Can you work these out from the model? Positions are in its coordinate system, mm. A direction names the side the tool comes from. Coordinates: 2 decimals unless noted, no trailing zeros. Order: outer loops, then holes, each group sorted by start corner. A loop starts at its lowest first (then second) coordinate and runs counter-clockwise, first axis right, second up. Notation, with made-up numbers: (-32, 55.25) -> (-26, 55.25) arc R22 ccw to (-26, 86.25) -> close; hole circle Ø11 at (2.5, -33). An arc over 180 degrees is marked (long way). Answer as a JSON object with one key per item and string values. Group by question number.
(1) Which directions (+Z, -Z, +X, -X, +Y, -Y) give clear straight access to the entire face, cutting with the end or side of a thin tool? Please do faces 5 (the cylindrical face through (-3, 0, 6)), 6 (the flat face through (5, 0, 4)), 7 (the flat face through (3, 1.5, 1)).
(2) For pin 1 (1 mm diameter, centred on x = 2, y = -1, fed in from +Z), with a flat end and sliding along its axis, tell me the tip position at first contact or that it passes through.
(3) If we mould it in two halves opening along X, with no side actions, what happens to faces 1 (the flat face through (2, 4, 4)), 2 (the flat face through (0, 0, 3)), 3 (the flat face through (-4, 0, 4)), 4 (the flat face through (9, 0, 6))? For each: pulls with the +X half, pulls with the -X half, needs draft (parallel to the pull), parting line crosses it, or undercut.
(4) I want a section at B-B, the plane x = 0. List the corners of the cut face in (y, z) for me, plus the area to 3 significant figures.
(5) I want a section at D-D, the plane z = 1. List the corners of the cut face in (x, y) for me, plus the area to 3 significant figures.
(6) I want a section at A-A, the plane z = 4. List the corners of the cut face in (x, y) for me.
(7) I want a section at C-C, the plane y = -2.5. List the corners of the cut face in (x, z) for me.
(8) I need wall thicknesses on line 1 (Y direction, x = 0, z = 5.2); line 2 (X direction, y = -0.25, z = 0.5); line 3 (Z direction, x = 5.25, y = -1.25). Which ranges of each line are inside material? Lowest first, please.
from build123d import *

# Parameters (mm, degrees)
SKETCH2_W           = 8
SKETCH2_H           = 8
BOSS_EXTRUDE1_DEPTH = 8
SKETCH3_R           = 3
CUT_EXTRUDE1_DEPTH  = 5
SKETCH5_W           = 8
SKETCH5_H           = 8
BOSS_EXTRUDE2_DEPTH = 5
SKETCH6_R           = 1.5
CUT_EXTRUDE2_DEPTH  = 4
CUT_EXTRUDE3_DEPTH  = 2.5
BOSS_EXTRUDE4_DEPTH = 2
CUT_EXTRUDE4_DEPTH  = 1
BOSS_EXTRUDE5_DEPTH = 2
SKETCH11_W          = 3
SKETCH11_H          = 3
CUT_EXTRUDE8_DEPTH  = 2.5


with BuildPart() as part:
    # Sketch2 → Boss-Extrude1 (new body)
    with BuildSketch(Plane.XY):
        Rectangle(SKETCH2_W, SKETCH2_H)
    extrude(amount=BOSS_EXTRUDE1_DEPTH)

    # Sketch3 → Cut-Extrude1 (cut)
    with BuildSketch(Plane.XY.offset(8)):
        Circle(SKETCH3_R)
    extrude(amount=-CUT_EXTRUDE1_DEPTH, mode=Mode.SUBTRACT)

    # Sketch5 → Boss-Extrude2 (add)
    with BuildSketch(Plane(origin=(4, 0, 0), x_dir=(0, 0, -1), z_dir=(1, 0, 0))):
        with Locations((-4, 0)):
            Rectangle(SKETCH5_W, SKETCH5_H)
    extrude(amount=BOSS_EXTRUDE2_DEPTH)

    # Sketch6 → Cut-Extrude2 (cut)
    with BuildSketch(Plane(origin=(9, 0, 0), x_dir=(0, 0, -1), z_dir=(1, 0, 0))):
        with Locations(Location((-4, 0, 0), (0, 0, 90))):
            Circle(SKETCH6_R)
    extrude(amount=-CUT_EXTRUDE2_DEPTH, mode=Mode.SUBTRACT)

    # Sketch7 → Cut-Extrude3 (cut)
    with BuildSketch(Plane(origin=(0, 0, 0), x_dir=(-1, 0, 0), z_dir=(0, 0, -1))):
        Polygon((-2.5, 2.121320344), (-0.378679656, 0), (-2.5, -2.121320344), (-4.621320344, 0), align=None)
    extrude(amount=-CUT_EXTRUDE3_DEPTH, mode=Mode.SUBTRACT)

    # Sketch8 → Boss-Extrude4 (add)
    with BuildSketch(Plane(origin=(0, 0, 0), x_dir=(-1, 0, 0), z_dir=(0, 0, -1))):
        Polygon((-4.621320344, 0), (-2.5, 2.121320344), (-0.378679656, 0), (-2.5, -2.121320344), align=None)
    extrude(amount=-BOSS_EXTRUDE4_DEPTH)

    # Sketch9 → Cut-Extrude4 (cut)
    with BuildSketch(Plane(origin=(0, 0, 0), x_dir=(-1, 0, 0), z_dir=(0, 0, -1))):
        Polygon((-6.487359326, 0), (-5.148694176, 2.68476733), (-2.463926846, 1.346102179), (-3.802591997, -1.338665151), align=None)
    extrude(amount=-CUT_EXTRUDE4_DEPTH, mode=Mode.SUBTRACT)

    # Sketch10 → Boss-Extrude5 (add)
    with BuildSketch(Plane(origin=(0, 0, 0), x_dir=(-1, 0, 0), z_dir=(0, 0, -1))):
        Polygon((-5.148694176, 2.68476733), (-2.463926846, 1.346102179), (-3.802591997, -1.338665151), (-6.487359326, 0), align=None)
    extrude(amount=-BOSS_EXTRUDE5_DEPTH)

    # Sketch11 → Cut-Extrude8 (cut)
    with BuildSketch(Plane(origin=(0, 0, 0), x_dir=(-1, 0, 0), z_dir=(0, 0, -1))):
        with Locations((-2.5, 0)):
            Rectangle(SKETCH11_W, SKETCH11_H)
    extrude(amount=-CUT_EXTRUDE8_DEPTH, mode=Mode.SUBTRACT)


solid = part.part
Computed values:
{
 "1": {"face 5": "+Z", "face 6": "+X", "face 7": "-Z"},
 "2": {"pin 1": "stops at z = 3"},
 "3": {"face 1": "needs draft", "face 2": "undercut", "face 3": "pulls with the -X half", "face 4": "pulls with the +X half"},
 "4": {"outline": "(-4, 0) -> (4, 0) -> (4, 8) -> (3, 8) -> (3, 3) -> (-3, 3) -> (-3, 8) -> (-4, 8) -> close", "area": "34.0 mm2"},
 "5": {"outline": "(-4, -4) -> (9, -4) -> (9, 4) -> (-4, 4) -> close; hole (1, -1.5) -> (4, -1.5) -> (4, 1.5) -> (1, 1.5) -> close", "area": "95.0 mm2"},
 "6": {"outline": "(-4, -4) -> (9, -4) -> (9, -1.5) -> (5, -1.5) -> (5, 1.5) -> (9, 1.5) -> (9, 4) -> (-4, 4) -> close; hole circle Ø6 at (0, 0)"},
 "7": {"outline": "(-4, 0) -> (9, 0) -> (9, 8) -> (1.66, 8) -> (1.66, 3) -> (-1.66, 3) -> (-1.66, 8) -> (-4, 8) -> close"},
 "8": {"line 1": "y = -4 to -3, 3 to 4", "line 2": "x = -4 to 1, 4 to 9", "line 3": "z = 0 to 3.17, 4.83 to 8"}
}
